CAD build for the part. Positions are in the model's coordinates, mm. Face numbers are marked on the shaded views. A direction names the side the tool comes from. Round coordinates to 2 decimals unless told otherwise and drop trailing zeros. Order: outer loops, then holes, each group sorted by start corner. A loop starts at its lowest first (then second) coordinate and runs counter-clockwise, first axis right, second up. Notation, with made-up numbers: M -27,-38 L 1,-38 A26 cw 1,-6 Z; hole C 82,41.5 d10. An arc over 180 degrees is marked long. Answer as a JSON object with one key per item and string values.
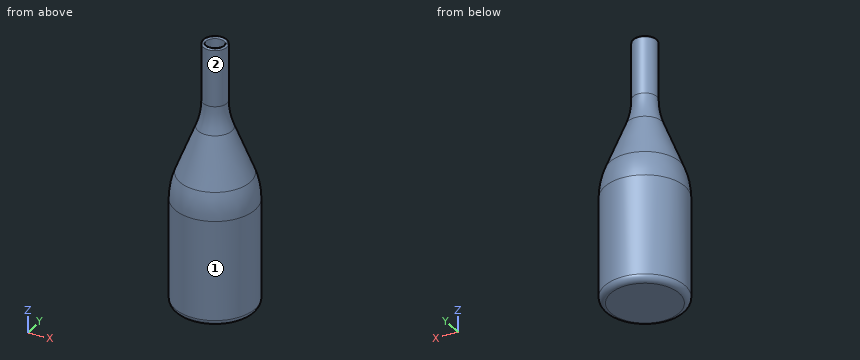
```python
from build123d import *

# Parameters (mm, degrees)
F2_R = 1.58749


# Not quite as in the source:
# - a fillet or chamfer is up to 0.001 mm smaller than in the source, because OpenCascade refuses the exact size


with BuildPart() as f1:
    # F0 (on Front) → F1 (revolve)
    with BuildSketch(Plane.XZ):
        with BuildLine():
            Line((12.7, 152.5613266138), (9.525, 152.5613266138))
            Line((9.525, 152.5613266138), (9.525, 90.8940221579))
            ThreePointArc((9.525, 90.8940221579), (10.9303408592, 76.0238211347), (15.0966000875, 61.6801763592))
            Line((15.0966000875, 61.6801763592), (34.5616279195, 12.5053692045))
            ThreePointArc((34.5616279195, 12.5053692045), (38.3945864095, -0.6907839889), (39.6875, -14.3713689303))
            Line((39.6875, -14.3713689303), (39.6875, -117.3136733862))
            ThreePointArc((39.6875, -117.3136733862), (37.8276280605, -121.8038014467), (33.3375, -123.6636733862))
            Line((33.3375, -123.6636733862), (0, -123.6636733862))
            Line((0, -123.6636733862), (0, -126.8386733862))
            Line((0, -126.8386733862), (36.5125, -126.8386733862))
            ThreePointArc((36.5125, -126.8386733862), (41.0026280605, -124.9788014467), (42.8625, -120.4886733862))
            Line((42.8625, -120.4886733862), (42.8625, -14.3713689303))
            ThreePointArc((42.8625, -14.3713689303), (41.5133727751, -0.095975948), (37.513763916, 13.6739230365))
            Line((37.513763916, 13.6739230365), (18.048736084, 62.8487301912))
            ThreePointArc((18.048736084, 62.8487301912), (14.0491272249, 76.6186291756), (12.7, 90.8940221579))
            Line((12.7, 90.8940221579), (12.7, 152.5613266138))
        make_face()
    revolve(axis=Axis((0, 0, 12.8613266138), (0, 0, -1)))

    # F2 (radius 1.5875 in the source; OpenCascade refuses exactly that, so slightly less here)
    f2_edges = [f1.edges().sort_by_distance(p)[0] for p in [
        (-12.7, 0, 152.561327),
        (-9.525, 0, 152.561327),
    ]]
    fillet(f2_edges, radius=F2_R)


solid = f1.part
```
Item 1: Drop flat-ended pins along their axis: pin 1 Ø3 at (x, z) = (10.5, 35.5) entering from -Y; pin 2 Ø12 at (x, z) = (-10.5, -47.5) entering from +Y; pin 3 Ø6 at (y, z) = (-17, 9.5) entering from -X. Give the stop position or say it passes through.
Worked answers:
{"pin 1": "stops at y = -27.74", "pin 2": "stops at y = 42.63", "pin 3": "stops at x = -36.81"}
Item 2: Saw through at B-B on z = 85.5. List the corners of the cut face in (x, y), and give its area (3 significant figures).
Worked answers:
{"outline": "C 0,0 d25.78; hole C 0,0 d19.42", "area": "226 mm2"}
Item 3: 3-axis set-ups, long thin cutter, end or side, ignore diameter. For the marked faces 1 and 2: which of +Z, -Z, +X, -X, +Y, -Y reach the whole face in a straight line?
Worked answers:
{"face 1": "+Z, -Z", "face 2": "+Z"}
Item 4: Saw through at A-A on z = -99. List the corners of the cut face in (x, y) (1 decimal), and give its area (3 significant figures).
Worked answers:
{"outline": "C 0,0 d85.7; hole C 0,0 d79.4", "area": "823 mm2"}
Item 5: Wall check: line 1 along X through (y, z) = (0, 117) (3 decimals); line 2 along X through (y, z) = (0, -62); line 3 along Y through (x, z) = (-30.5, -66). Give the ranges that are in metal, low to high. Write a range as [from, to].
Worked answers:
{"line 1": "x = [-12.7, -9.525], [9.525, 12.7]", "line 2": "x = [-42.86, -39.69], [39.69, 42.86]", "line 3": "y = [-30.12, -25.39], [25.39, 30.12]"}
